Could you check a few things on this model? Use its own coordinates, in mm. Face numbers are marked on the shaded views. Round coordinates to 2 decimals unless told otherwise and drop trailing zeros. Loops run counter-clockwise (first coordinate to the right, second up) from the corner with the lowest first, then second, coordinate; pieces in that order, holes last. Notation, with made-up numbers: (21.5, -4.75) -> (70.5, -4.75) arc R17 ccw to (70.5, 7.25) -> close; hole circle Ø11 at (-15, 11). An arc over 180 degrees is marked (long way). Write each question's results on one line, items separated by ' | '.
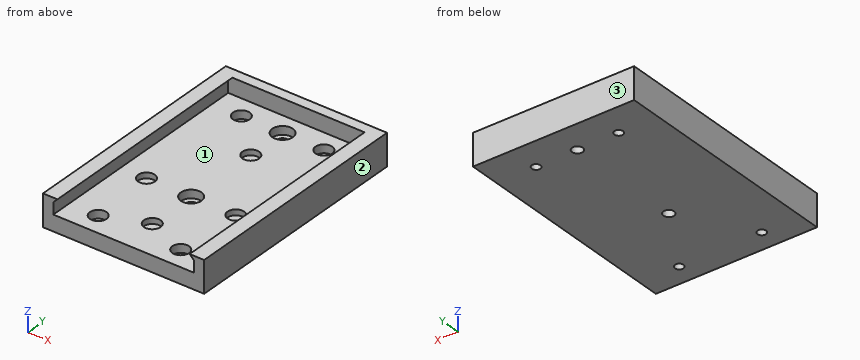
from build123d import *

# Parameters (mm, degrees)
SKETCH1_W                = 68.1
SKETCH1_H                = 110
SKETCH1_R                = 2.1
SKETCH1_R_2              = 4.05
SKETCH1_R_3              = 2.6
BOSS_EXTRUDE1_DEPTH      = 7.7
SKETCH2_R                = 6.304633146
SKETCH2_R_2              = 7.334333348
SKETCH2_R_3              = 8.114040952
SKETCH2_R_4              = 11.073656437
BOSS_EXTRUDE2_DEPTH      = 5
SKETCH3_R                = 4.05
SKETCH3_R_2              = 5
CUT_EXTRUDE1_DEPTH       = 4
SKETCH4_W                = 68.1
SKETCH4_H                = 5
BOSS_EXTRUDE3_DEPTH      = 7.7
BOSS_EXTRUDE3_DEPTH_BACK = 7.7
BOSS_EXTRUDE4_DEPTH      = 115


with BuildPart() as part:
    # Sketch1 → Boss-Extrude1 (new body)
    with BuildSketch(Plane.XY):
        Rectangle(SKETCH1_W, SKETCH1_H)
        with Locations((20, 45)):
            Circle(SKETCH1_R, mode=Mode.SUBTRACT)
        with Locations((-20, 45)):
            Circle(SKETCH1_R, mode=Mode.SUBTRACT)
        with Locations((20, -45)):
            Circle(SKETCH1_R, mode=Mode.SUBTRACT)
        with Locations((-20, -45)):
            Circle(SKETCH1_R, mode=Mode.SUBTRACT)
        with Locations((21.650635095, -12.5)):
            Circle(SKETCH1_R_2, mode=Mode.SUBTRACT)
        with Locations((0, 25)):
            Circle(SKETCH1_R_2, mode=Mode.SUBTRACT)
        with Locations((-21.650635095, -12.5)):
            Circle(SKETCH1_R_2, mode=Mode.SUBTRACT)
        with Locations((0, -36.95)):
            Circle(SKETCH1_R_2, mode=Mode.SUBTRACT)
        with Locations((0, 45)):
            Circle(SKETCH1_R_3, mode=Mode.SUBTRACT)
        with Locations((0, -12.5)):
            Circle(SKETCH1_R_3, mode=Mode.SUBTRACT)
    extrude(amount=BOSS_EXTRUDE1_DEPTH)

    # Sketch2 → Boss-Extrude2 (add)
    with BuildSketch(Plane(origin=(0, 0, 0), x_dir=(-1, 0, 0), z_dir=(0, 0, -1))):
        with Locations((-21.650635095, -12.5)):
            Circle(SKETCH2_R)
        with Locations((0, 25)):
            Circle(SKETCH2_R_2)
        with Locations((21.650635095, -12.5)):
            Circle(SKETCH2_R_3)
        with Locations((0, -36.95)):
            Circle(SKETCH2_R_4)
    extrude(amount=-BOSS_EXTRUDE2_DEPTH)

    # Sketch3 → Cut-Extrude1 (cut)
    with BuildSketch(Plane(origin=(0, 0, 7.7), x_dir=(-1, 0, 0), z_dir=(0, 0, -1))):
        with Locations((-20, 45)):
            Circle(SKETCH3_R)
        with Locations((20, 45)):
            Circle(SKETCH3_R)
        with Locations((-20, -45)):
            Circle(SKETCH3_R)
        with Locations((20, -45)):
            Circle(SKETCH3_R)
        with Locations((0, 45)):
            Circle(SKETCH3_R_2)
        with Locations((0, -12.5)):
            Circle(SKETCH3_R_2)
    extrude(amount=CUT_EXTRUDE1_DEPTH, mode=Mode.SUBTRACT)

    # Sketch4 → Boss-Extrude3 (add, two sides)
    with BuildSketch(Plane.XY.offset(7.7)) as boss_extrude3_sk:
        with Locations((0, 57.5)):
            Rectangle(SKETCH4_W, SKETCH4_H)
    extrude(amount=BOSS_EXTRUDE3_DEPTH)
    extrude(boss_extrude3_sk.sketch, amount=-BOSS_EXTRUDE3_DEPTH_BACK)

    # Sketch7 → Boss-Extrude4 (add)
    with BuildSketch(Plane.XZ.offset(55)):
        Polygon((-34.05, 15.4), (-32.05, 15.4), (-34.05, 13.4), (-34.05, 0), (-39.05, 0), (-39.05, 15.4), align=None)
        Polygon((39.05, 0), (34.05, 0), (34.05, 13.4), (32.05, 15.4), (34.05, 15.4), (39.05, 15.4), align=None)
    extrude(amount=-BOSS_EXTRUDE4_DEPTH)


solid = part.part
1) I'm going to push flat-ended pins straight in: pin 1 (4 mm diameter, centred on x = -19, y = -46.5, fed in from +Z); pin 2 (13 mm diameter, centred on x = 0, y = 25, fed in from +Z); pin 3 (3.5 mm diameter, centred on x = -20, y = 45, fed in from -Z); pin 4 (6 mm diameter, centred on x = 13, z = 13, fed in from -Y). Where does each tip first touch, or does it pass through?
Model answer:
pin 1: stops at z = 3.7 | pin 2: stops at z = 7.7 | pin 3: passes through | pin 4: stops at y = 55
2) I want a section at D-D, the plane z = 11. Write out the boundary of the cut face in (x, y), plus the area to 3 significant figures.
Model answer:
outline: (-39.05, -55) -> (-34.05, -55) -> (-34.05, 55) -> (34.05, 55) -> (34.05, -55) -> (39.05, -55) -> (39.05, 60) -> (-39.05, 60) -> close | area: 1,490 mm2
3) I want a section at C-C, the plane y = -45. Write out the boundary of the cut face in (x, z).
Model answer:
outline: (-39.05, 0) -> (-22.1, 0) -> (-22.1, 3.7) -> (-24.05, 3.7) -> (-24.05, 7.7) -> (-34.05, 7.7) -> (-34.05, 13.4) -> (-32.05, 15.4) -> (-39.05, 15.4) -> close; (-17.9, 0) -> (17.9, 0) -> (17.9, 3.7) -> (15.95, 3.7) -> (15.95, 7.7) -> (-15.95, 7.7) -> (-15.95, 3.7) -> (-17.9, 3.7) -> close; (22.1, 0) -> (39.05, 0) -> (39.05, 15.4) -> (32.05, 15.4) -> (34.05, 13.4) -> (34.05, 7.7) -> (24.05, 7.7) -> (24.05, 3.7) -> (22.1, 3.7) -> close
4) If we mould it in two halves opening along X, with no side actions, what happens to the marked faces 1, 2 and 3? For each: released by +X, released by -X, zero draft, split by the parting line, or undercut.
Model answer:
face 1: undercut | face 2: released by +X | face 3: zero draft
5) I want a section at B-B, the plane x = 0. Give the number of separate pieces and of enclosed holes in the cut face, plus the area to 3 significant figures.
Model answer:
separate pieces: 3 | enclosed holes: 0 | area: 762 mm2
6) I want a section at A-A, the plane y = -12.5. Write out the boundary of the cut face in (x, z).
Model answer:
outline: (-39.05, 0) -> (-2.6, 0) -> (-2.6, 3.7) -> (-5, 3.7) -> (-5, 7.7) -> (-17.6, 7.7) -> (-17.6, 5) -> (-25.7, 5) -> (-25.7, 7.7) -> (-34.05, 7.7) -> (-34.05, 13.4) -> (-32.05, 15.4) -> (-39.05, 15.4) -> close; (2.6, 0) -> (39.05, 0) -> (39.05, 15.4) -> (32.05, 15.4) -> (34.05, 13.4) -> (34.05, 7.7) -> (25.7, 7.7) -> (25.7, 5) -> (17.6, 5) -> (17.6, 7.7) -> (5, 7.7) -> (5, 3.7) -> (2.6, 3.7) -> close
7) I need wall thicknesses on line 1 (Y direction, x = 20, z = 2.5); line 2 (Y direction, x = 0, z = 6.05); line 3 (X direction, y = 5.5, z = 12). Which ranges of each line are inside material? Lowest first, please.
Model answer:
line 1: y = -55 to -47.1, -42.9 to 42.9, 47.1 to 60 | line 2: y = -55 to -41, -32.9 to -17.5, -7.5 to 20.95, 29.05 to 40, 50 to 60 | line 3: x = -39.05 to -34.05, 34.05 to 39.05
